```python
from build123d import *

# Parameters (mm, degrees)
SKETCH1_W           = 250
SKETCH1_H           = 283
SKETCH1_R           = 2.3
SKETCH1_W_2         = 20
SKETCH1_H_2         = 4.8
BOSS_EXTRUDE1_DEPTH = 5
SKETCH2_W           = 5
SKETCH2_H           = 20
BOSS_EXTRUDE2_DEPTH = 5
SKETCH3_R           = 2.1
SKETCH3_W           = 28
SKETCH3_H           = 20
CUT_EXTRUDE1_DEPTH  = 5
SKETCH4_W           = 20
SKETCH4_H           = 30
CUT_EXTRUDE2_DEPTH  = 5
SKETCH5_R           = 2.1
CUT_EXTRUDE3_DEPTH  = 6
SKETCH6_R           = 2.1
CUT_EXTRUDE4_DEPTH  = 5
SKETCH7_R           = 2.1
CUT_EXTRUDE5_DEPTH  = 5


with BuildPart() as part:
    # Sketch1 → Boss-Extrude1 (new body)
    with BuildSketch(Plane.XY):
        with Locations((125, 136.5)):
            Rectangle(SKETCH1_W, SKETCH1_H)
        with Locations((125, 125.1)):
            Circle(SKETCH1_R, mode=Mode.SUBTRACT)
        with Locations((125, 205.1)):
            Circle(SKETCH1_R, mode=Mode.SUBTRACT)
        with Locations((60, 2.5)):
            Rectangle(SKETCH1_W_2, SKETCH1_H_2, mode=Mode.SUBTRACT)
        with Locations((190, 2.5)):
            Rectangle(SKETCH1_W_2, SKETCH1_H_2, mode=Mode.SUBTRACT)
        with Locations((190, 270.5)):
            Rectangle(SKETCH1_W_2, SKETCH1_H_2, mode=Mode.SUBTRACT)
        with Locations((60, 270.5)):
            Rectangle(SKETCH1_W_2, SKETCH1_H_2, mode=Mode.SUBTRACT)
    extrude(amount=BOSS_EXTRUDE1_DEPTH)

    # Sketch2 → Boss-Extrude2 (add)
    with BuildSketch(Plane.XY.offset(5)):
        with Locations((-2.5, 198)):
            Rectangle(SKETCH2_W, SKETCH2_H)
        with Locations((-2.5, 75)):
            Rectangle(SKETCH2_W, SKETCH2_H)
        with Locations((252.5, 198)):
            Rectangle(SKETCH2_W, SKETCH2_H)
        with Locations((252.5, 75)):
            Rectangle(SKETCH2_W, SKETCH2_H)
    extrude(amount=-BOSS_EXTRUDE2_DEPTH)

    # Sketch3 → Cut-Extrude1 (cut)
    with BuildSketch(Plane.XY.offset(5)):
        with Locations((190, 85)):
            Circle(SKETCH3_R)
        with Locations((230, 85)):
            Circle(SKETCH3_R)
        with Locations((210, 85)):
            Rectangle(SKETCH3_W, SKETCH3_H)
    extrude(amount=-CUT_EXTRUDE1_DEPTH, mode=Mode.SUBTRACT)

    # Sketch4 → Cut-Extrude2 (cut)
    with BuildSketch(Plane.XY.offset(5)):
        with Locations((86.25, 35.2)):
            Rectangle(SKETCH4_W, SKETCH4_H)
    extrude(amount=-CUT_EXTRUDE2_DEPTH, mode=Mode.SUBTRACT)

    # Sketch5 → Cut-Extrude3 (cut, through all)
    with BuildSketch(Plane.XY.offset(5)):
        with Locations((98.18627451, 15.72)):
            Circle(SKETCH5_R)
        with Locations((74.31372549, 15.72)):
            Circle(SKETCH5_R)
        with Locations((74.31372549, 54.68)):
            Circle(SKETCH5_R)
        with Locations((98.18627451, 54.68)):
            Circle(SKETCH5_R)
    extrude(amount=-CUT_EXTRUDE3_DEPTH, mode=Mode.SUBTRACT)

    # Sketch6 → Cut-Extrude4 (cut)
    with BuildSketch(Plane.XY.offset(5)):
        with Locations((235, 253)):
            Circle(SKETCH6_R)
        with Locations((15, 253)):
            Circle(SKETCH6_R)
    extrude(amount=-CUT_EXTRUDE4_DEPTH, mode=Mode.SUBTRACT)

    # Sketch7 → Cut-Extrude5 (cut)
    with BuildSketch(Plane.XY.offset(5)):
        with Locations((15, 105)):
            Circle(SKETCH7_R)
        with Locations((235, 105)):
            Circle(SKETCH7_R)
    extrude(amount=-CUT_EXTRUDE5_DEPTH, mode=Mode.SUBTRACT)


solid = part.part
```
Input: part model. Units: mm. Frame: model coordinates. Give positions to 0.01 mm unless a question says otherwise; leave off trailing zeros. Order: outer loops, then holes, each group sorted by start corner. A loop starts at its lowest first (then second) coordinate and runs counter-clockwise, first axis right, second up. Notation, with made-up numbers: M 2,83.25 L 17,83.25 A23 cw 17,100.25 Z; hole C 23.5,9 d5. An arc over 180 degrees is marked long. One line per question, with ' | ' between items.
1) Contact query for flat-ended pins moving along their axis: P1, Ø2.5, axis at x = -1.5, z = 2, coming from the -Y side; P2, Ø5, axis at x = 235, y = 105, coming from the +Z side; P3, Ø2, axis at y = 33.5, z = 2.5, coming from the +X side; P4, Ø2.5, axis at y = 271.5, z = 3.5, coming from the -X side. Output: stop coordinate, or through.
Filled in:
P1: stops at y = 65 | P2: stops at z = 5 | P3: stops at x = 250 | P4: stops at x = 0
2) Ray query, L1, parallel to X at y = 253, z = 3.95; L2, parallel to Y at x = 60, z = 2.8; L3, parallel to Y at x = 15, z = 1.2. Return the intervals inside material, ascending.
Filled in:
L1: x = 0 to 12.9, 17.1 to 232.9, 237.1 to 250 | L2: y = -5 to 0.1, 4.9 to 268.1, 272.9 to 278 | L3: y = -5 to 102.9, 107.1 to 250.9, 255.1 to 278
3) Section C-C on y = 131. Output: boundary loops of the cut face in (x, z), and give its area (3 significant figures).
Filled in:
outline: M 0,0 L 250,0 L 250,5 L 0,5 Z | area: 1,250 mm2
4) Section B-B on z = 1.65. State how many separate pieces and enclosed holes the cut face has, and give its area (3 significant figures).
Filled in:
separate pieces: 1 | enclosed holes: 18 | area: 69,400 mm2
5) Section A-A on x = 82. Output: boundary loops of the cut face in (y, z).
Filled in:
outline: M -5,0 L 20.2,0 L 20.2,5 L -5,5 Z; M 50.2,0 L 278,0 L 278,5 L 50.2,5 Z
